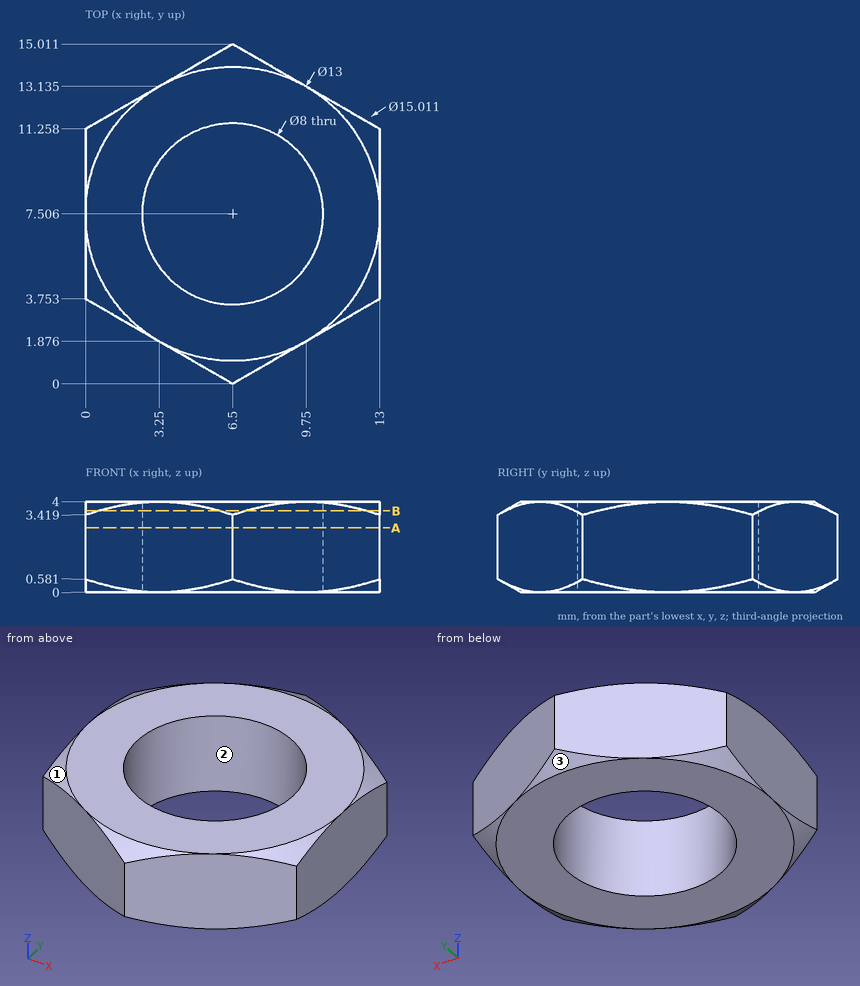
Print and shaded views of the part. All mm, measured from the part's lowest x, y and z. Coordinates: 2 decimals unless noted, no trailing zeros. Loops run counter-clockwise (first coordinate to the right, second up) from the corner with the lowest first, then second, coordinate; pieces in that order, holes last. Notation, with made-up numbers: (-24.5, 42) - (7.5, 42) arc R20 ccw to (7.5, 79) - close; hole circle Ø3 at (79.5, 73.5). An arc over 180 degrees is marked (long way). Write item = value, one per line. Start each with the question number.
Item 1: Saw through at A-A, the plane z = 2.85. List the corners of the cut face in (x, y) (1 decimal).
Item 2: Saw through at B-B, the plane z = 3.6. List the corners of the cut face in (x, y) (1 decimal).
Item 3: Drop flat-ended pins along their axis: pin 1 Ø1 at (y, z) = (3, 3) entering from +X; pin 2 Ø1 at (y, z) = (8.5, 3) entering from -X. Give the stop position or say it passes through.
Item 4: Wall check: probe 1 along X at (y, z) = (7.5, 3.3); probe 2 along X at (y, z) = (8.25, 0.35); probe 3 along Y at (x, z) = (5, 0.4) (1 decimal). Give the ranges that are in metal, low to high. Write a range as [from, to].
Item 5: Pull direction Y, two halves, no side cores. Call the marked faces 1, 2 and 3: +Y half, -Y half, draft (parallel to the pull), parting line (faces both ways), or undercut.
Answers:
q1.outline = (0, 3.8) - (6.5, 0) - (13, 3.8) - (13, 11.3) - (6.5, 15) - (0, 11.3) - close; hole circle Ø8 at (6.5, 7.5)
q2.outline = (0, 4.4) arc R7.2 ccw to (0.6, 3.4) - (5.9, 0.3) arc R7.2 ccw to (7.1, 0.3) - (12.4, 3.4) arc R7.2 ccw to (13, 4.4) - (13, 10.6) arc R7.2 ccw to (12.4, 11.6) - (7.1, 14.7) arc R7.2 ccw to (5.9, 14.7) - (0.6, 11.6) arc R7.2 ccw to (0, 10.6) - close; hole circle Ø8 at (6.5, 7.5)
q3.pin_1 = 12.56
q3.pin_2 = 0
q4.probe_1 = [0, 2.5], [10.5, 13]
q4.probe_2 = [0, 2.57], [10.43, 13]
q4.probe_3 = [0.9, 3.8], [11.2, 14.1]
q5.face_1 = -Y half
q5.face_2 = undercut
q5.face_3 = +Y half
